Input: dimensioned drawing with shaded views. Units: mm. Origin: part minimum x, y, z. Coordinates: 2 decimals unless noted, no trailing zeros. Loops run counter-clockwise (first coordinate to the right, second up) from the corner with the lowest first, then second, coordinate; pieces in that order, holes last.
(1) Section C-C, the plane z = 5. Return loops of the section in (x, y), then the cut area to 3 significant figures.
(2) Contact query for flat-ended pins moving along their axis: P1, Ø1.5, axis at x = 49.5, y = 0.5, coming from the -Z side; P2, Ø3, axis at x = 57, z = 5, coming from the -Y side; P3, Ø1, axis at y = 1.5, z = 8.5, coming from the -X side. Output: stop coordinate, or through.
(3) Section A-A, the plane z = 9. Return loops of the section in (x, y).
(4) Section D-D, the plane y = 0.9. Return loops of the section in (x, z), then the cut area to 3 significant figures.
(5) Section B-B, the plane x = 5. Return loops of the section in (y, z), then the cut area to 3 significant figures.
(6) Line query: L1, parallel to X at y = 1.3, z = 5; L2, parallel to X at y = 2.2, z = 4; L3, parallel to Z at x = 5, y = 1.85. Output: solid intervals per line, ascending.
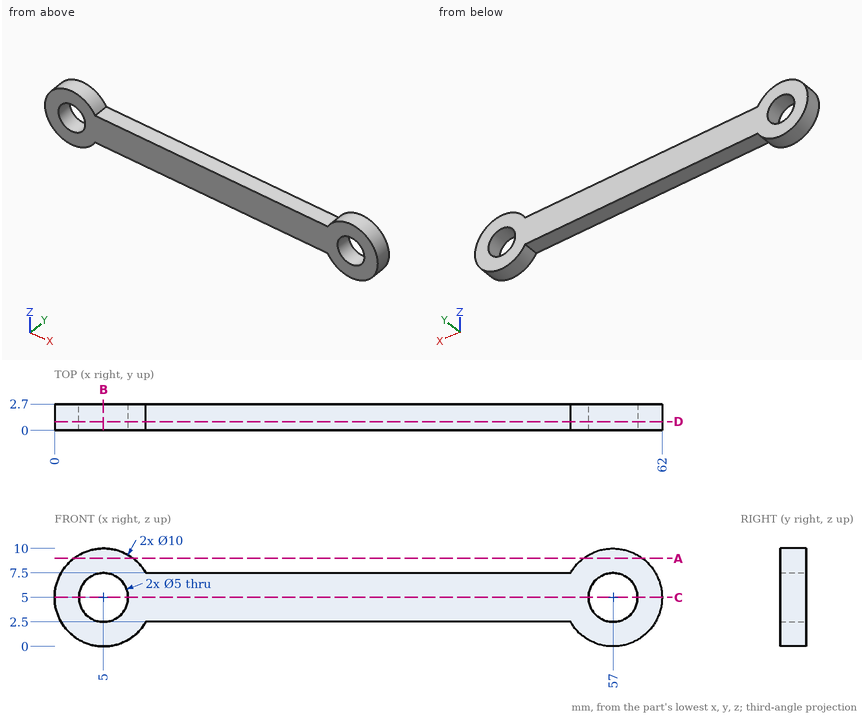
Report:
1. outline: (0, 0) - (2.5, 0) - (2.5, 2.7) - (0, 2.7) - close; (7.5, 0) - (54.5, 0) - (54.5, 2.7) - (7.5, 2.7) - close; (59.5, 0) - (62, 0) - (62, 2.7) - (59.5, 2.7) - close
1. area: 140 mm2
2. P1: stops at z = 2.5
2. P2: passes through
2. P3: stops at x = 1
3. outline: (2, 0) - (8, 0) - (8, 2.7) - (2, 2.7) - close; (54, 0) - (60, 0) - (60, 2.7) - (54, 2.7) - close
4. outline: (9.33, 2.5) - (52.67, 2.5) arc R5 ccw (long way) to (52.67, 7.5) - (9.33, 7.5) arc R5 ccw (long way) to start; hole circle Ø5 at (5, 5); hole circle Ø5 at (57, 5)
4. area: 330 mm2
5. outline: (0, 0) - (2.7, 0) - (2.7, 2.5) - (0, 2.5) - close; (0, 7.5) - (2.7, 7.5) - (2.7, 10) - (0, 10) - close
5. area: 13.5 mm2
6. L1: x = 0 to 2.5, 7.5 to 54.5, 59.5 to 62
6. L2: x = 0.1 to 2.71, 7.29 to 54.71, 59.29 to 61.9
6. L3: z = 0 to 2.5, 7.5 to 10
